from build123d import *

# Parameters (mm, degrees)
F0_R     = 9.6
F0_R_2   = 2.1
F1_DEPTH = 2.5
F3_DEPTH = 6
F4_R     = 2.1
F5_DEPTH = 6
F6_SIZE  = 0.3
F7_SIZE  = 0.2
F8_SIZE  = 0.2


with BuildPart() as f1:
    # F0 (on Top) → F1 (new body)
    with BuildSketch(Plane.XY):
        Circle(F0_R)
        Circle(F0_R_2, mode=Mode.SUBTRACT)
    extrude(amount=-F1_DEPTH)

    # F2 (on face) → F3 (join)
    with BuildSketch(Plane(origin=(0, 0, -2.5), x_dir=(1, 0, 0), z_dir=(0, 0, -1))):
        with BuildLine():
            Line((-3.889087, -3.889087), (-6.010408, -6.010408))
            ThreePointArc((-6.010408, -6.010408), (-3.252809, -7.852976), (0, -8.5))
            Line((0, -8.5), (0, -5.5))
            ThreePointArc((0, -5.5), (-2.104759, -5.081337), (-3.889087, -3.889087))
        make_face()
    extrude(amount=F3_DEPTH)

    # F4 (on face) → F5 (join)
    with BuildSketch(Plane.XY):
        with BuildLine():
            ThreePointArc((-3.11127, 3.11127), (-3.516618, 3.176372), (-3.926339, 3.202339))
            ThreePointArc((-3.926339, 3.202339), (-4.019657, 3.084391), (-4.109433, 2.963726))
            ThreePointArc((-4.109433, 2.963726), (-3.978308, 2.574687), (-3.810512, 2.2))
            ThreePointArc((-3.810512, 2.2), (-3.717923, 2.097301), (-3.617501, 2.002248))
            Line((-3.617501, 2.002248), (-3.179227, 1.749211))
            ThreePointArc((-3.179227, 1.749211), (-2.878815, 2.208992), (-2.512452, 2.618168))
            Line((-2.512452, 2.618168), (-2.870301, 2.976017))
            ThreePointArc((-2.870301, 2.976017), (-2.988107, 3.048416), (-3.11127, 3.11127))
        make_face()
        with BuildLine():
            ThreePointArc((-1.878686, 3.104474), (-2.208992, 2.878815), (-2.512452, 2.618168))
            ThreePointArc((-2.512452, 2.618168), (-2.878815, 2.208992), (-3.179227, 1.749211))
            ThreePointArc((-3.179227, 1.749211), (-3.352451, 1.388631), (-3.484932, 1.011174))
            ThreePointArc((-3.484932, 1.011174), (-3.597623, 0.473636), (-3.627897, -0.074753))
            ThreePointArc((-3.627897, -0.074753), (-3.597623, -0.473636), (-3.523626, -0.866763))
            ThreePointArc((-3.523626, -0.866763), (-3.352451, -1.388631), (-3.104474, -1.878686))
            ThreePointArc((-3.104474, -1.878686), (-2.878815, -2.208992), (-2.618168, -2.512452))
            ThreePointArc((-2.618168, -2.512452), (-2.208992, -2.878815), (-1.749211, -3.179227))
            ThreePointArc((-1.749211, -3.179227), (-1.388631, -3.352451), (-1.011174, -3.484932))
            ThreePointArc((-1.011174, -3.484932), (-0.473636, -3.597623), (0.074753, -3.627897))
            ThreePointArc((0.074753, -3.627897), (0.473636, -3.597623), (0.866763, -3.523626))
            ThreePointArc((0.866763, -3.523626), (1.388631, -3.352451), (1.878686, -3.104474))
            ThreePointArc((1.878686, -3.104474), (2.208992, -2.878815), (2.512452, -2.618168))
            ThreePointArc((2.512452, -2.618168), (2.878815, -2.208992), (3.179227, -1.749211))
            ThreePointArc((3.179227, -1.749211), (3.352451, -1.388631), (3.484932, -1.011174))
            ThreePointArc((3.484932, -1.011174), (3.592553, -0.510669), (3.628667, 0))
            ThreePointArc((3.628667, 0), (3.628474, 0.037378), (3.627897, 0.074753))
            ThreePointArc((3.627897, 0.074753), (3.597623, 0.473636), (3.523626, 0.866763))
            ThreePointArc((3.523626, 0.866763), (3.352451, 1.388631), (3.104474, 1.878686))
            ThreePointArc((3.104474, 1.878686), (2.878815, 2.208992), (2.618168, 2.512452))
            ThreePointArc((2.618168, 2.512452), (2.208992, 2.878815), (1.749211, 3.179227))
            ThreePointArc((1.749211, 3.179227), (1.388631, 3.352451), (1.011174, 3.484932))
            ThreePointArc((1.011174, 3.484932), (0.473636, 3.597623), (-0.074753, 3.627897))
            ThreePointArc((-0.074753, 3.627897), (-0.473636, 3.597623), (-0.866763, 3.523626))
            ThreePointArc((-0.866763, 3.523626), (-1.388631, 3.352451), (-1.878686, 3.104474))
        make_face()
        Circle(F4_R, mode=Mode.SUBTRACT)
        with BuildLine():
            Line((-2.131723, 3.542748), (-1.878686, 3.104474))
            ThreePointArc((-1.878686, 3.104474), (-1.388631, 3.352451), (-0.866763, 3.523626))
            Line((-0.866763, 3.523626), (-0.997745, 4.012457))
            ThreePointArc((-0.997745, 4.012457), (-1.063568, 4.134059), (-1.138804, 4.250074))
            ThreePointArc((-1.138804, 4.250074), (-1.457294, 4.509128), (-1.79914, 4.736476))
            ThreePointArc((-1.79914, 4.736476), (-1.938929, 4.68099), (-2.07701, 4.621378))
            ThreePointArc((-2.07701, 4.621378), (-2.157972, 4.218898), (-2.2, 3.810512))
            ThreePointArc((-2.2, 3.810512), (-2.171165, 3.675278), (-2.131723, 3.542748))
        make_face()
        with BuildLine():
            ThreePointArc((-3.627897, -0.074753), (-3.597623, 0.473636), (-3.484932, 1.011174))
            Line((-3.484932, 1.011174), (-3.973763, 1.142156))
            ThreePointArc((-3.973763, 1.142156), (-4.111985, 1.145953), (-4.250074, 1.138804))
            ThreePointArc((-4.250074, 1.138804), (-4.633667, 0.99251), (-5.001479, 0.810137))
            ThreePointArc((-5.001479, 0.810137), (-5.023321, 0.661333), (-5.040736, 0.511946))
            ThreePointArc((-5.040736, 0.511946), (-4.732659, 0.24059), (-4.4, 0))
            ThreePointArc((-4.4, 0), (-4.268466, -0.042645), (-4.133972, -0.074753))
            Line((-4.133972, -0.074753), (-3.627897, -0.074753))
        make_face()
        with BuildLine():
            Line((-0.074753, 4.133972), (-0.074753, 3.627897))
            ThreePointArc((-0.074753, 3.627897), (0.473636, 3.597623), (1.011174, 3.484932))
            Line((1.011174, 3.484932), (1.142156, 3.973763))
            ThreePointArc((1.142156, 3.973763), (1.145953, 4.111985), (1.138804, 4.250074))
            ThreePointArc((1.138804, 4.250074), (0.99251, 4.633667), (0.810137, 5.001479))
            ThreePointArc((0.810137, 5.001479), (0.661333, 5.023321), (0.511946, 5.040736))
            ThreePointArc((0.511946, 5.040736), (0.24059, 4.732659), (0, 4.4))
            ThreePointArc((0, 4.4), (-0.042645, 4.268466), (-0.074753, 4.133972))
        make_face()
        with BuildLine():
            ThreePointArc((-3.104474, -1.878686), (-3.352451, -1.388631), (-3.523626, -0.866763))
            Line((-3.523626, -0.866763), (-4.012457, -0.997745))
            ThreePointArc((-4.012457, -0.997745), (-4.134059, -1.063568), (-4.250074, -1.138804))
            ThreePointArc((-4.250074, -1.138804), (-4.509128, -1.457294), (-4.736476, -1.79914))
            ThreePointArc((-4.736476, -1.79914), (-4.68099, -1.938929), (-4.621378, -2.07701))
            ThreePointArc((-4.621378, -2.07701), (-4.218898, -2.157972), (-3.810512, -2.2))
            ThreePointArc((-3.810512, -2.2), (-3.675278, -2.171165), (-3.542748, -2.131723))
            Line((-3.542748, -2.131723), (-3.104474, -1.878686))
        make_face()
        with BuildLine():
            Line((2.002248, 3.617501), (1.749211, 3.179227))
            ThreePointArc((1.749211, 3.179227), (2.208992, 2.878815), (2.618168, 2.512452))
            Line((2.618168, 2.512452), (2.976017, 2.870301))
            ThreePointArc((2.976017, 2.870301), (3.048416, 2.988107), (3.11127, 3.11127))
            ThreePointArc((3.11127, 3.11127), (3.176372, 3.516618), (3.202339, 3.926339))
            ThreePointArc((3.202339, 3.926339), (3.084391, 4.019657), (2.963726, 4.109433))
            ThreePointArc((2.963726, 4.109433), (2.574687, 3.978308), (2.2, 3.810512))
            ThreePointArc((2.2, 3.810512), (2.097301, 3.717923), (2.002248, 3.617501))
        make_face()
        with BuildLine():
            ThreePointArc((-1.749211, -3.179227), (-2.208992, -2.878815), (-2.618168, -2.512452))
            Line((-2.618168, -2.512452), (-2.976017, -2.870301))
            ThreePointArc((-2.976017, -2.870301), (-3.048416, -2.988107), (-3.11127, -3.11127))
            ThreePointArc((-3.11127, -3.11127), (-3.176372, -3.516618), (-3.202339, -3.926339))
            ThreePointArc((-3.202339, -3.926339), (-3.084391, -4.019657), (-2.963726, -4.109433))
            ThreePointArc((-2.963726, -4.109433), (-2.574687, -3.978308), (-2.2, -3.810512))
            ThreePointArc((-2.2, -3.810512), (-2.097301, -3.717923), (-2.002248, -3.617501))
            Line((-2.002248, -3.617501), (-1.749211, -3.179227))
        make_face()
        with BuildLine():
            Line((3.542748, 2.131723), (3.104474, 1.878686))
            ThreePointArc((3.104474, 1.878686), (3.352451, 1.388631), (3.523626, 0.866763))
            Line((3.523626, 0.866763), (4.012457, 0.997745))
            ThreePointArc((4.012457, 0.997745), (4.134059, 1.063568), (4.250074, 1.138804))
            ThreePointArc((4.250074, 1.138804), (4.509128, 1.457294), (4.736476, 1.79914))
            ThreePointArc((4.736476, 1.79914), (4.68099, 1.938929), (4.621378, 2.07701))
            ThreePointArc((4.621378, 2.07701), (4.218898, 2.157972), (3.810512, 2.2))
            ThreePointArc((3.810512, 2.2), (3.675278, 2.171165), (3.542748, 2.131723))
        make_face()
        with BuildLine():
            ThreePointArc((0.074753, -3.627897), (-0.473636, -3.597623), (-1.011174, -3.484932))
            Line((-1.011174, -3.484932), (-1.142156, -3.973763))
            ThreePointArc((-1.142156, -3.973763), (-1.145953, -4.111985), (-1.138804, -4.250074))
            ThreePointArc((-1.138804, -4.250074), (-0.99251, -4.633667), (-0.810137, -5.001479))
            ThreePointArc((-0.810137, -5.001479), (-0.661333, -5.023321), (-0.511946, -5.040736))
            ThreePointArc((-0.511946, -5.040736), (-0.24059, -4.732659), (0, -4.4))
            ThreePointArc((0, -4.4), (0.042645, -4.268466), (0.074753, -4.133972))
            Line((0.074753, -4.133972), (0.074753, -3.627897))
        make_face()
        with BuildLine():
            Line((4.133972, 0.074753), (3.627897, 0.074753))
            ThreePointArc((3.627897, 0.074753), (3.628474, 0.037378), (3.628667, 0))
            ThreePointArc((3.628667, 0), (3.592553, -0.510669), (3.484932, -1.011174))
            Line((3.484932, -1.011174), (3.973763, -1.142156))
            ThreePointArc((3.973763, -1.142156), (4.111985, -1.145953), (4.250074, -1.138804))
            ThreePointArc((4.250074, -1.138804), (4.633667, -0.99251), (5.001479, -0.810137))
            ThreePointArc((5.001479, -0.810137), (5.023321, -0.661333), (5.040736, -0.511946))
            ThreePointArc((5.040736, -0.511946), (4.732659, -0.24059), (4.4, 0))
            ThreePointArc((4.4, 0), (4.268466, 0.042645), (4.133972, 0.074753))
        make_face()
        with BuildLine():
            ThreePointArc((1.878686, -3.104474), (1.388631, -3.352451), (0.866763, -3.523626))
            Line((0.866763, -3.523626), (0.997745, -4.012457))
            ThreePointArc((0.997745, -4.012457), (1.063568, -4.134059), (1.138804, -4.250074))
            ThreePointArc((1.138804, -4.250074), (1.457294, -4.509128), (1.79914, -4.736476))
            ThreePointArc((1.79914, -4.736476), (1.938929, -4.68099), (2.07701, -4.621378))
            ThreePointArc((2.07701, -4.621378), (2.157972, -4.218898), (2.2, -3.810512))
            ThreePointArc((2.2, -3.810512), (2.171165, -3.675278), (2.131723, -3.542748))
            Line((2.131723, -3.542748), (1.878686, -3.104474))
        make_face()
        with BuildLine():
            ThreePointArc((3.179227, -1.749211), (2.878815, -2.208992), (2.512452, -2.618168))
            Line((2.512452, -2.618168), (2.870301, -2.976017))
            ThreePointArc((2.870301, -2.976017), (2.988107, -3.048416), (3.11127, -3.11127))
            ThreePointArc((3.11127, -3.11127), (3.516618, -3.176372), (3.926339, -3.202339))
            ThreePointArc((3.926339, -3.202339), (4.019657, -3.084391), (4.109433, -2.963726))
            ThreePointArc((4.109433, -2.963726), (3.978308, -2.574687), (3.810512, -2.2))
            ThreePointArc((3.810512, -2.2), (3.717923, -2.097301), (3.617501, -2.002248))
            Line((3.617501, -2.002248), (3.179227, -1.749211))
        make_face()
    extrude(amount=F5_DEPTH)

    # F6
    f6_edges = [f1.edges().sort_by_distance(p)[0] for p in [
        (-2.1, 0, -2.5),
    ]]
    chamfer(f6_edges, length=F6_SIZE)

    # F7
    f7_edges = [f1.edges().sort_by_distance(p)[0] for p in [
        (-2.1, 0, 6),
    ]]
    chamfer(f7_edges, length=F7_SIZE)

    # F8
    f8_edges = [f1.edges().sort_by_distance(p)[0] for p in [
        (-9.6, 0, -2.5),
        (-9.6, 0, 0),
    ]]
    chamfer(f8_edges, length=F8_SIZE)


solid = f1.part
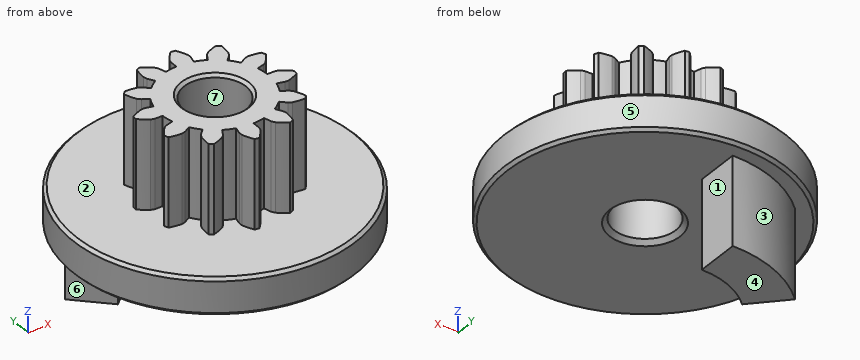
Input: part model. Units: mm. Frame: model coordinates. Face numbers are marked on the shaded views. A direction names the side the tool comes from. Coordinates: 2 decimals unless noted, no trailing zeros. Order: outer loops, then holes, each group sorted by start corner. A loop starts at its lowest first (then second) coordinate and runs counter-clockwise, first axis right, second up. Notation, with made-up numbers: M 0,-3.75 L 21,-3.75 A22 ccw 21,7.25 Z; hole C 45,54 d7. An arc over 180 degrees is marked long. Answer in a Markdown table with one row per item.
(1) Draft query along X for the marked faces 4, 5, 6 and 7. Return one class per face: pulls with the +X half, pulls with the -X half, needs draft (parallel to the pull), parting line crosses it, or undercut.
Numbers:
| item | result |
|---|---|
| face 4 | needs draft |
| face 5 | parting line crosses it |
| face 6 | pulls with the -X half |
| face 7 | undercut |
(2) Material intervals for line 1 (Z direction, x = 4.25, y = 3); line 2 (Y direction, x = 3.25, z = 4); line 3 (Z direction, x = 3.25, y = 0), sorted ascending. Write a range as [from, to].
Numbers:
| item | result |
|---|---|
| line 1 | z = [-2.5, 0] |
| line 2 | y = [-3.14, -1.79], [-1.61, 1.96] |
| line 3 | z = [-2.5, 6] |
(3) Access query for the marked faces 1, 2 and 3. Directions: +Z, -Z, +X, -X, +Y, -Y. A direction counts if a zero-diameter tool reaches every point of the face in a straight line with its end or side. Return the directions, or none.
Numbers:
| item | result |
|---|---|
| face 1 | -Z, +X, +Y, -Y |
| face 2 | +Z |
| face 3 | -Z, -X, +Y |
(4) Section query B-B, the plane z = -0.5. Output: boundary loops of the cut face in (x, y), plus the area to 3 significant figures.
Numbers:
| item | result |
|---|---|
| outline | C 0,0 d19.2; hole C 0,0 d4.2 |
| area | 276 mm^2 |
(5) Section query A-A, the plane z = -7.5. Output: boundary loops of the cut face in (x, y).
Numbers:
| item | result |
|---|---|
| outline | M -6.01,6.01 L -3.89,3.89 A5.5 cw 0,5.5 L 0,8.5 A8.5 ccw Z |
(6) Contact query for flat-ended pins moving along their axis: pin 1 Ø1 at (x, y) = (7.5, -6.5) entering from -Z; pin 2 Ø2 at (x, y) = (-5, 4) entering from +Z; pin 3 Ø4 at (x, y) = (0, 0) entering from -Z; pin 4 Ø0.6 at (y, z) = (4, 4) entering from -X. Output: stop coordinate, or through.
Numbers:
| item | result |
|---|---|
| pin 1 | stops at z = -2.48 |
| pin 2 | stops at z = 0 |
| pin 3 | passes through |
| pin 4 | stops at x = -2.2 |
